Verification items for this drawing (mm, ordinates from the low corner). A direction names the side the tool comes from. Round coordinates to 2 decimals unless told otherwise and drop trailing zeros. Loops run counter-clockwise (first coordinate to the right, second up) from the corner with the lowest first, then second, coordinate; pieces in that order, holes last. Notation, with made-up numbers: (-40, 12.25) -> (-25, 12.25) arc R25 cw to (-25, 47.25) -> close; hole circle Ø1 at (77, 22.5). An arc over 180 degrees is marked (long way). Use a Markdown table: item, result. Add a question column.
Q1. Gauge pin test, flat ends, axial feed: P1, Ø2, axis at x = 10, y = 2, coming from the -Z side; P2, Ø3, axis at x = 11, z = 8.5, coming from the -Y side; P3, Ø0.8, axis at y = 3, z = 11, coming from the -X side; P4, Ø1.5, axis at x = 6.5, y = 19, coming from the -Z side. Record the tip position at first contact, or that the pin passes through.
Q2. Set-up check for the marked faces 4, 5 and 6: record each of +Z, -Z, +X, -X, +Y, -Y from which the full face is reachable in a straight line by a thin tool's end or side.
Q3. Release check for a two-part mould opening along Y. For the marked faces 1, 2 and 3 record: released by +Y, released by -Y, zero draft, split by the parting line, or undercut.
Q4. Sectioned sample at D-D, the plane z = 9. Enter the section's corners in (x, y), then the cut area to 3 significant figures.
Q5. Material ranges on L1, parallel to Y at x = 10.16, z = 9.75; L2, parallel to X at y = 13.75, z = 8.5; L3, parallel to Y at x = 8.75, z = 9.75, recorded low to high.
Q6. Sectioned sample at B-B, the plane x = 14. Enter the section's corners in (y, z), then the cut area to 3 significant figures.
Q7. Sectioned sample at C-C, the plane z = 11.5. Enter the section's corners in (x, y).
Q8. Sectioned sample at A-A, the plane y = 13.97. Enter the section's corners in (x, z).
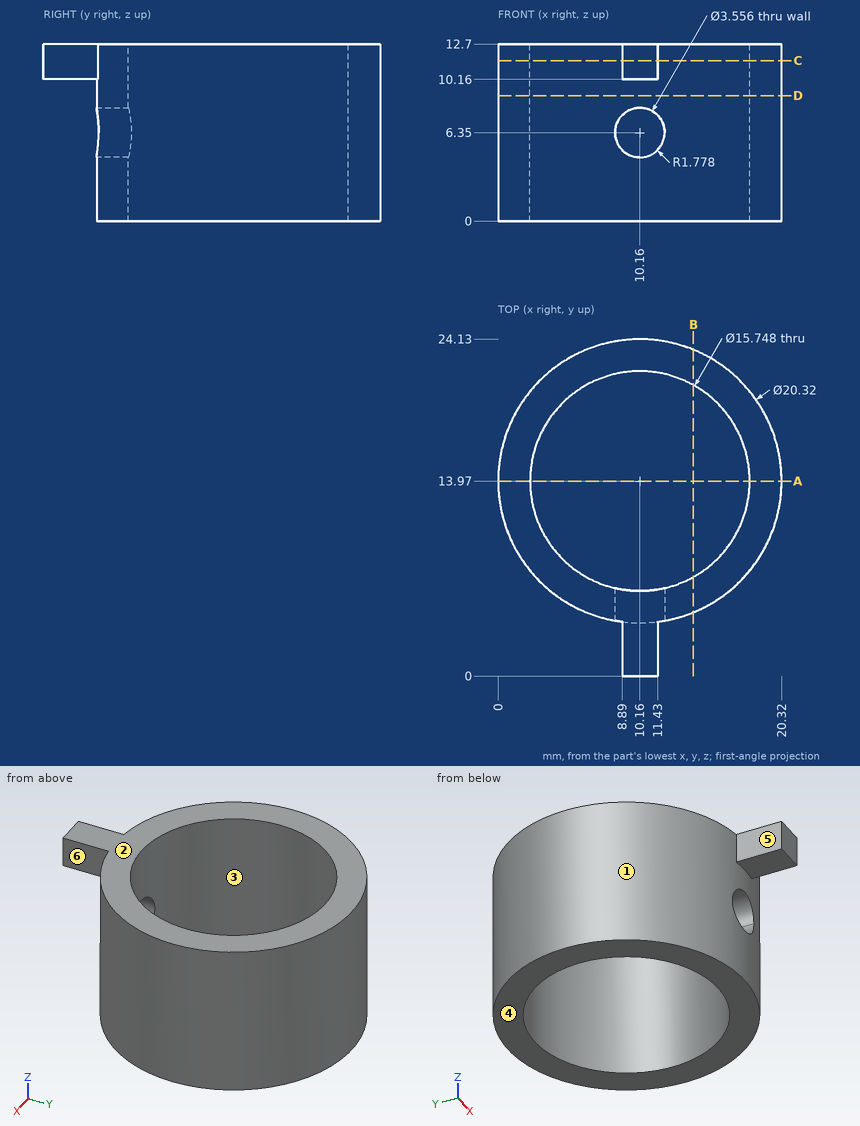
Values:
| question | item | result |
|---|---|---|
| 1 | P1 | z = 10.16 |
| 1 | P2 | y = 3.81 |
| 1 | P3 | x = 8.89 |
| 1 | P4 | through |
| 2 | face 4 | -Z, +X, -X, +Y, -Y |
| 2 | face 5 | +Z, -Z, -X, -Y |
| 2 | face 6 | +Z, -Z, +X, -Y |
| 3 | face 1 | split by the parting line |
| 3 | face 2 | zero draft |
| 3 | face 3 | undercut |
| 4 | outline | circle Ø20.32 at (10.16, 13.97); hole circle Ø15.75 at (10.16, 13.97) |
| 4 | area | 130 mm^2 |
| 5 | L1 | 3.81 to 6.1, 21.84 to 24.13 |
| 5 | L2 | 0 to 2.29, 18.03 to 20.32 |
| 5 | L3 | 3.91 to 6.22, 21.72 to 24.03 |
| 6 | outline | (4.56, 0) -> (7.1, 0) -> (7.1, 12.7) -> (4.56, 12.7) -> close; (20.84, 0) -> (23.38, 0) -> (23.38, 12.7) -> (20.84, 12.7) -> close |
| 6 | area | 64.3 mm^2 |
| 7 | outline | (8.89, 0) -> (11.43, 0) -> (11.43, 3.89) arc R10.16 ccw (long way) to (8.89, 3.89) -> close; hole circle Ø15.75 at (10.16, 13.97) |
| 8 | outline | (0, 0) -> (2.29, 0) -> (2.29, 12.7) -> (0, 12.7) -> close; (18.03, 0) -> (20.32, 0) -> (20.32, 12.7) -> (18.03, 12.7) -> close |
